Answer from the drawing. Dimensions are ordinates in mm from the lowest x, y and z of the part. Round coordinates to 2 decimals unless told otherwise and drop trailing zeros. Loops run counter-clockwise (first coordinate to the right, second up) from the corner with the lowest first, then second, coordinate; pieces in that order, holes last.
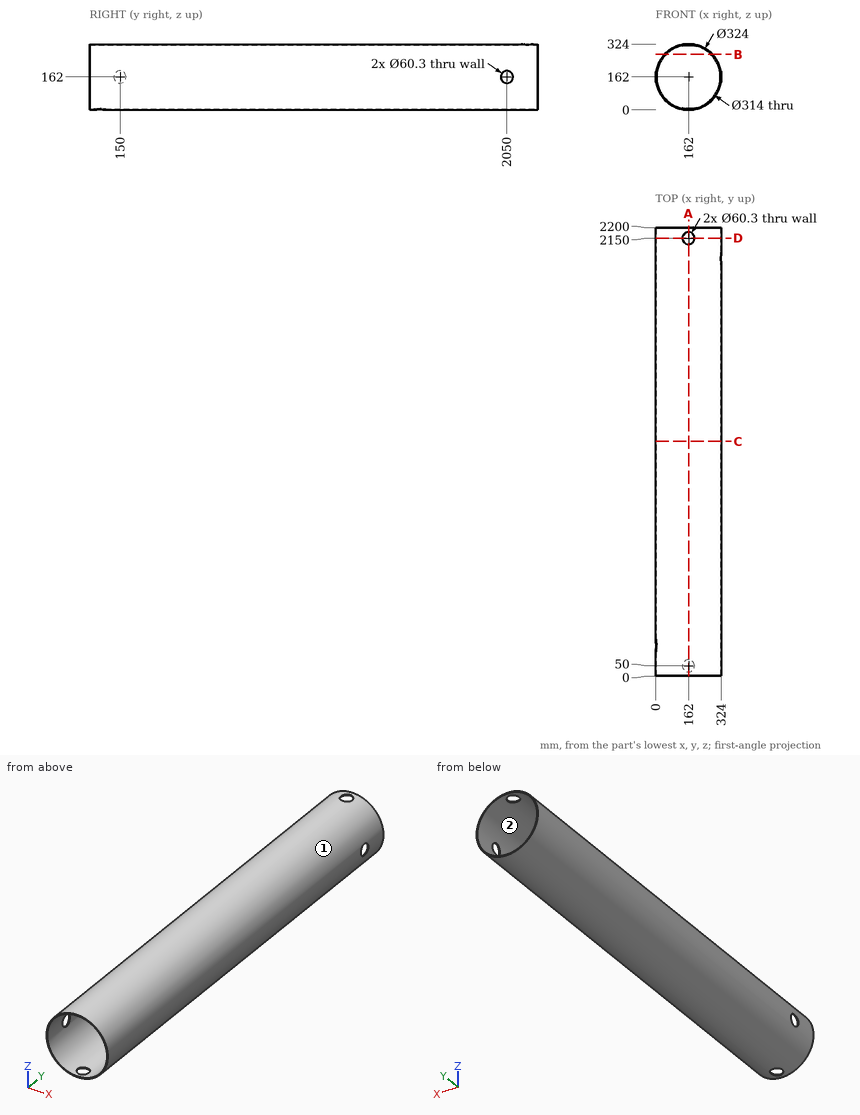
1. Find section B-B (z = 272.5). Write down the section's boundary in (x, y), then the cut area to 3 significant figures.
Answer key:
outline: (43.54, 0) - (50.47, 0) - (50.47, 2200) - (43.54, 2200) - close; (273.53, 0) - (280.46, 0) - (280.46, 2200) - (273.53, 2200) - close
area: 30,500 mm2
2. Find section A-A (x = 162). Write down the section's boundary in (y, z), then the cut area to 3 significant figures.
Answer key:
outline: (0, 0) - (19.85, 0) - (19.85, 5) - (0, 5) - close; (0, 319) - (2119.85, 319) - (2119.85, 324) - (0, 324) - close; (80.15, 0) - (2200, 0) - (2200, 5) - (80.15, 5) - close; (2180.15, 319) - (2200, 319) - (2200, 324) - (2180.15, 324) - close
area: 21,400 mm2
3. Consider probe 1 along Z at (x, y) = (162, 990.5); probe 2 along Z at (x, y) = (156.5, 1079); probe 3 along X at (y, z) = (1552.5, 173.5). Determine where each line is inside the solid, lowest interval first.
Answer key:
probe 1: z = 0 to 5, 319 to 324
probe 2: z = 0.09 to 5.1, 318.9 to 323.91
probe 3: x = 0.41 to 5.42, 318.58 to 323.59
4. Find section D-D (y = 2150). Write down the section's boundary in (x, z), then the cut area to 3 significant figures.
Answer key:
outline: (131.85, 316.08) - (131.85, 321.17) arc R162 ccw (long way) to (192.15, 321.17) - (192.15, 316.08) arc R157 cw (long way) to start
area: 4,710 mm2
5. Find section C-C (y = 1152). Write down the section's boundary in (x, z), then the cut area to 3 significant figures.
Answer key:
outline: circle Ø324 at (162, 162); hole circle Ø314 at (162, 162)
area: 5,010 mm2
6. Given pin 1 (8 mm diameter, centred on x = 72, y = 792.5, fed in from +Z); pin 2 (10 mm diameter, centred on x = 220.5, y = 647.5, fed in from -Z); pin 3 (6 mm diameter, centred on x = 154.5, y = 1134.5, fed in from -Z), each flat-ended and moving along its own axis, determine where each tip first touches the part or whether it passes through.
Answer key:
pin 1: stops at z = 299.29
pin 2: stops at z = 9.09
pin 3: stops at z = 0.06
7. Determine the mould class of the marked faces 1 and 2 for opening direction X: +X half, -X half, draft (parallel to the pull), parting line (faces both ways), or undercut.
Answer key:
face 1: parting line
face 2: undercut
